```python
from build123d import *

# Parameters (mm, degrees)
BOSS_EXTRUDE1_DEPTH       = 5
FILLET3_RADIUS            = 10
FILLET3_LENGTH            = 5
FILLET4_RADIUS            = 10
FILLET4_LENGTH            = 5
FILLET2_R                 = 2
LAYER_FIX_HOLE_DEPTH      = 229.869504303
LAYER_FIX_HOLE_DEPTH_BACK = 229.869504303
SKETCH2_R                 = 1.6
SKETCH3_R                 = 1.6
ARM_FIX_HOLE_DEPTH        = 229.869504303
SKETCH4_W                 = 15.5
SKETCH4_H                 = 2.5
IR_FIX_HOLE_DEPTH         = 229.869504303
CHAMFER1_SIZE             = 3
SKETCH5_W                 = 15.5
SKETCH5_H                 = 2.5
BOSS_EXTRUDE2_DEPTH       = 5
TURN_ON_OFF_SWITCH_REACH  = 230.87
SKETCH6_W                 = 13
SKETCH6_H                 = 8
CUT_EXTRUDE2_DEPTH        = 229.869504303
CUT_EXTRUDE2_DEPTH_BACK   = 229.869504303
SKETCH9_R                 = 1.7
SKETCH9_W                 = 45
SKETCH9_H                 = 5


with BuildPart() as part:
    # Sketch1 → Boss-Extrude1 (new body)
    with BuildSketch(Plane(origin=(0, 0, 0), x_dir=(1, 0, 0), z_dir=(0, 1, 0))):
        Polygon((-117.5, -110), (117.5, -110), (117.5, -90), (107.5, -90), (107.5, -20), (117.5, -20), (117.5, 100), (107.5, 100), (107.5, 170), (127.5, 170), (127.5, 190), (-127.5, 190), (-127.5, 170), (-107.5, 170), (-107.5, 100), (-117.5, 100), (-117.5, -20), (-107.5, -20), (-107.5, -90), (-117.5, -90), align=None)
    extrude(amount=BOSS_EXTRUDE1_DEPTH)

    # Fillet3: full round fillet: the end face becomes a half cylinder, R = half its width
    fillet3_face = Plane((127.5, 2.5, -180), x_dir=(0, 1, 0), z_dir=(1, 0, 0))  # on the end face: x along it, z out of the body
    fillet3_slab = fillet3_face.offset(-FILLET3_RADIUS / 2) * Box(FILLET3_LENGTH, 2 * FILLET3_RADIUS, FILLET3_RADIUS, mode=Mode.PRIVATE)  # the body's end, R deep
    fillet3_round = Plane((117.5, 2.5, -180), x_dir=(1, 0, 0), z_dir=(0, 1, 0)) * Cylinder(FILLET3_RADIUS, FILLET3_LENGTH, mode=Mode.PRIVATE)  # its axis R under the face
    add(fillet3_slab - fillet3_round, mode=Mode.SUBTRACT)

    # Fillet4: full round fillet: the end face becomes a half cylinder, R = half its width
    fillet4_face = Plane((-127.5, 2.5, -180), x_dir=(0, 1, 0), z_dir=(-1, 0, 0))  # on the end face: x along it, z out of the body
    fillet4_slab = fillet4_face.offset(-FILLET4_RADIUS / 2) * Box(FILLET4_LENGTH, 2 * FILLET4_RADIUS, FILLET4_RADIUS, mode=Mode.PRIVATE)  # the body's end, R deep
    fillet4_round = Plane((-117.5, 2.5, -180), x_dir=(-1, 0, 0), z_dir=(0, 1, 0)) * Cylinder(FILLET4_RADIUS, FILLET4_LENGTH, mode=Mode.PRIVATE)  # its axis R under the face
    add(fillet4_slab - fillet4_round, mode=Mode.SUBTRACT)

    # Fillet2
    fillet2_edges = [part.edges().sort_by_distance(p)[0] for p in [
        (117.5, 2.5, 110),
        (-117.5, 2.5, 110),
        (-107.5, 2.5, 90),
        (-107.5, 2.5, 20),
        (-107.5, 2.5, -100),
        (-107.5, 2.5, -170),
        (107.5, 2.5, -170),
        (107.5, 2.5, -100),
        (107.5, 2.5, 20),
        (107.5, 2.5, 90),
    ]]
    fillet(fillet2_edges, radius=FILLET2_R)

    # Sketch2 → layer fix hole (cut, two sides: drawn at the far end of the back side and taken through both)
    with BuildSketch(Plane(origin=(0, 5, 0), x_dir=(1, 0, 0), z_dir=(0, 1, 0)).offset(-LAYER_FIX_HOLE_DEPTH_BACK)):
        with Locations(Location((107.5, 180, 0), (0, 0, 270))):
            Circle(SKETCH2_R)
        with Locations(Location((107.5, 40, 0), (0, 0, 270))):
            Circle(SKETCH2_R)
        with Locations(Location((107.5, -99, 0), (0, 0, 270))):
            Circle(SKETCH2_R)
        with Locations(Location((-107.5, 40, 0), (0, 0, 270))):
            Circle(SKETCH2_R)
        with Locations(Location((-107.5, -99, 0), (0, 0, 270))):
            Circle(SKETCH2_R)
        with Locations(Location((-107.5, 180, 0), (0, 0, 270))):
            Circle(SKETCH2_R)
        with Locations(Location((0, -99, 0), (0, 0, 270))):
            Circle(SKETCH2_R)
        with Locations(Location((55, -99, 0), (0, 0, 270))):
            Circle(SKETCH2_R)
        with Locations(Location((-55, -99, 0), (0, 0, 270))):
            Circle(SKETCH2_R)
        with Locations(Location((-107.5, 90, 0), (0, 0, 270))):
            Circle(SKETCH2_R)
        with Locations(Location((107.5, 90, 0), (0, 0, 270))):
            Circle(SKETCH2_R)
        with Locations(Location((-107.5, -10, 0), (0, 0, 270))):
            Circle(SKETCH2_R)
        with Locations(Location((107.5, -10, 0), (0, 0, 270))):
            Circle(SKETCH2_R)
    extrude(amount=LAYER_FIX_HOLE_DEPTH + LAYER_FIX_HOLE_DEPTH_BACK, mode=Mode.SUBTRACT)

    # Sketch3 → arm fix hole (cut, through all)
    with BuildSketch(Plane(origin=(0, 5, 0), x_dir=(1, 0, 0), z_dir=(0, 1, 0))):
        with Locations(Location((44, 110.5, 0), (0, 0, 270))):
            Circle(SKETCH3_R)
        with Locations(Location((44, 69.5, 0), (0, 0, 270))):
            Circle(SKETCH3_R)
        with Locations(Location((-44, 69.5, 0), (0, 0, 270))):
            Circle(SKETCH3_R)
        with Locations(Location((-44, 110.5, 0), (0, 0, 270))):
            Circle(SKETCH3_R)
        with BuildLine():
            Line((-39.597979746, 92.828427125), (-2.828427125, 129.597979746))
            ThreePointArc((-2.828427125, 129.597979746), (0, 130.769552622), (2.828427125, 129.597979746))
            Line((2.828427125, 129.597979746), (39.597979746, 92.828427125))
            ThreePointArc((39.597979746, 92.828427125), (40.769552622, 90), (39.597979746, 87.171572875))
            Line((39.597979746, 87.171572875), (2.828427125, 50.402020254))
            ThreePointArc((2.828427125, 50.402020254), (0, 49.230447378), (-2.828427125, 50.402020254))
            Line((-2.828427125, 50.402020254), (-39.597979746, 87.171572875))
            ThreePointArc((-39.597979746, 87.171572875), (-40.769552622, 90), (-39.597979746, 92.828427125))
        make_face()
    extrude(amount=-ARM_FIX_HOLE_DEPTH, mode=Mode.SUBTRACT)

    # Sketch4 → IR fix hole (cut, through all)
    with BuildSketch(Plane(origin=(0, 5, 0), x_dir=(1, 0, 0), z_dir=(0, 1, 0))):
        with Locations((-25, 184.75)):
            Rectangle(SKETCH4_W, SKETCH4_H)
        with Locations((-65, 184.75)):
            Rectangle(SKETCH4_W, SKETCH4_H)
        with Locations((5, 184.75)):
            Rectangle(SKETCH4_W, SKETCH4_H)
        with Locations((35, 184.75)):
            Rectangle(SKETCH4_W, SKETCH4_H)
    extrude(amount=-IR_FIX_HOLE_DEPTH, mode=Mode.SUBTRACT)

    # Chamfer1
    chamfer1_edges = [part.edges().sort_by_distance(p)[0] for p in [
        (-117.5, 2.5, 90),
        (-117.5, 2.5, 20),
        (-117.5, 2.5, -100),
        (117.5, 2.5, -100),
        (117.5, 2.5, 20),
        (117.5, 2.5, 90),
    ]]
    chamfer(chamfer1_edges, length=CHAMFER1_SIZE)

    # Sketch5 → Boss-Extrude2 (add)
    with BuildSketch(Plane(origin=(0, 5, 0), x_dir=(1, 0, 0), z_dir=(0, 1, 0))):
        with Locations((-65, 184.75)):
            Rectangle(SKETCH5_W, SKETCH5_H)
    extrude(amount=-BOSS_EXTRUDE2_DEPTH)

    # Sketch6 → Turn on_off Switch (cut, up to next)
    with BuildSketch(Plane(origin=(0, 5, 0), x_dir=(1, 0, 0), z_dir=(0, 1, 0)), mode=Mode.PRIVATE) as turn_on_off_switch_sk1:
        Rectangle(SKETCH6_W, SKETCH6_H)
    turn_on_off_switch_tool1 = extrude(turn_on_off_switch_sk1.sketch, amount=-TURN_ON_OFF_SWITCH_REACH, mode=Mode.PRIVATE) & part.part
    add(turn_on_off_switch_tool1.solids().sort_by_distance((0, 5, 0))[0], mode=Mode.SUBTRACT)

    # Sketch9 → Cut-Extrude2 (cut, two sides: drawn at the far end of the back side and taken through both)
    with BuildSketch(Plane(origin=(0, 5, 0), x_dir=(1, 0, 0), z_dir=(0, 1, 0)).offset(-CUT_EXTRUDE2_DEPTH_BACK)):
        with Locations(Location((-37.25, 177.35, 0), (0, 0, 90))):
            Circle(SKETCH9_R)
        with Locations(Location((37.25, 177.35, 0), (0, 0, 270))):
            Circle(SKETCH9_R)
        with Locations(Location((37.25, 146.85, 0), (0, 0, 90))):
            Circle(SKETCH9_R)
        with Locations(Location((-37.25, 146.85, 0), (0, 0, 270))):
            Circle(SKETCH9_R)
        with Locations((12.5, 146.7)):
            Rectangle(SKETCH9_W, SKETCH9_H)
    extrude(amount=CUT_EXTRUDE2_DEPTH + CUT_EXTRUDE2_DEPTH_BACK, mode=Mode.SUBTRACT)


solid = part.part
```
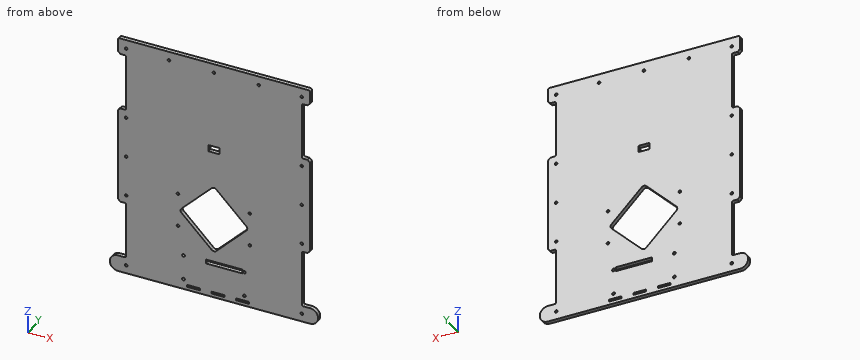
Verification items for the finished model (mm, model axes). Round coordinates to 2 decimals unless told otherwise and drop trailing zeros. Write each question's results on one line, items separated by ' | '. Start each with the question number.
1. Depth check by flat-ended pin: P1, Ø5, axis at x = -55, z = 99, coming from the -Y side; P2, Ø1.5, axis at y = 2.5, z = -147, coming from the +X side; P3, Ø1.2, axis at y = 2.5, z = -184.5, coming from the +X side; P4, Ø3, axis at y = 2.5, z = 5.5, coming from the -X side. Enter the tip coordinate at first touch or a pass-through.
2. Material ranges on probe 1 along X at (y, z) = (1.85, 99); probe 2 along X at (y, z) = (2.55, -146.85); probe 3 along Z at (x, y) = (0, 2.25), recorded low to high. Write a range as from..to.
3. Cross-section at A-A (y = 2.15). Count the separate pieces of the cut face and the enclosed holes in it, then the cut area to 3 significant figures.
Solutions:
1) P1: stops at y = 0 | P2: stops at x = 107.5 | P3: stops at x = 126.71 | P4: stops at x = -117.5
2) probe 1: x = -117.5..-109.1, -105.9..-56.6, -53.4..-1.6, 1.6..53.4, 56.6..105.9, 109.1..117.5 | probe 2: x = -107.5..-38.95, -35.55..-10, 35..35.55, 38.95..107.5 | probe 3: z = -190..-186, -183.5..-149.2, -144.2..-130.77, -49.23..-4, 4..97.4, 100.6..110
3) separate pieces: 1 | enclosed holes: 27 | area: 63,800 mm2
